Read the model definition and answer for the solid it produces. Units are mm, in the model's axes. Face numbers are marked on the shaded views. A direction names the side the tool comes from. Coordinates: 2 decimals unless noted, no trailing zeros. Order: outer loops, then holes, each group sorted by start corner. A loop starts at its lowest first (then second) coordinate and runs counter-clockwise, first axis right, second up. Notation, with made-up numbers: (-10, -2.5) - (42, -2.5) arc R14 cw to (42, 12.5) - close; hole circle Ø6 at (14, -19). An arc over 180 degrees is marked (long way). Use one line per item in the form item = value.
```python
from build123d import *

# Parameters (mm, degrees)
F0_W     = 40
F0_H     = 26
F1_DEPTH = 17
F2_T     = -1.5
F3_W     = 37
F3_H     = 8.5
F4_DEPTH = 2
F5_W     = 8.4
F5_H     = 3.5
F6_DEPTH = 1.5
F7_SIZE  = 2
F8_R     = 5


with BuildPart() as f1:
    # F0 (on Top) → F1 (new body)
    with BuildSketch(Plane.XY):
        Rectangle(F0_W, F0_H)
    extrude(amount=F1_DEPTH)

    # F2
    f2_openings = [f1.faces().sort_by_distance(p)[0] for p in [
        (0, 0, 17),
    ]]
    offset(amount=F2_T, openings=f2_openings)

    # F3 (on face) → F4 (join)
    with BuildSketch(Plane.XY.offset(1.5)):
        Rectangle(F3_W, F3_H)
    extrude(amount=F4_DEPTH)

    # F5 (on face) → F6 (cut, through all)
    with BuildSketch(Plane.YZ.offset(20)):
        with Locations((0, 5.25)):
            Rectangle(F5_W, F5_H)
    extrude(amount=-F6_DEPTH, mode=Mode.SUBTRACT)

    # F7
    f7_edges = [f1.edges().sort_by_distance(p)[0] for p in [
        (-18.5, 11.5, 9.25),
        (18.5, 11.5, 9.25),
        (18.5, -11.5, 9.25),
        (-18.5, -11.5, 9.25),
    ]]
    chamfer(f7_edges, length=F7_SIZE)

    # F8
    f8_edges = [f1.edges().sort_by_distance(p)[0] for p in [
        (-20, 13, 8.5),
        (20, 13, 8.5),
        (20, -13, 8.5),
        (-20, -13, 8.5),
    ]]
    fillet(f8_edges, radius=F8_R)


solid = f1.part
```
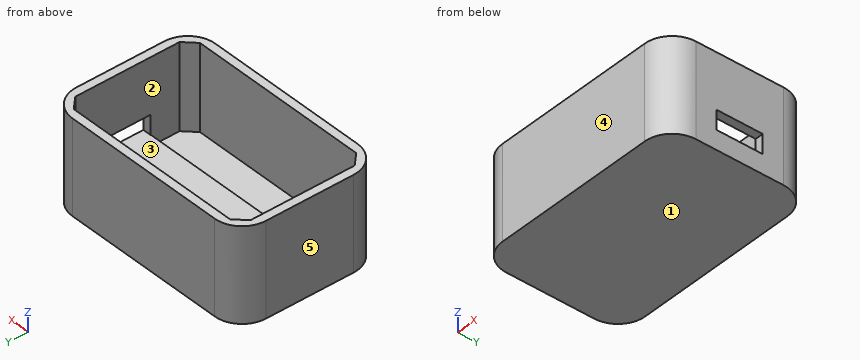
(1) Section D-D, the plane x = 7 is taken. Write down the section's boundary in (y, z).
Answer list:
outline = (-13, 0) - (13, 0) - (13, 17) - (11.5, 17) - (11.5, 1.5) - (4.25, 1.5) - (4.25, 3.5) - (-4.25, 3.5) - (-4.25, 1.5) - (-11.5, 1.5) - (-11.5, 17) - (-13, 17) - close
(2) Given pin 1 Ø1.5 at (x, y) = (13, 3.5) entering from +Z; pin 2 Ø3.5 at (x, y) = (9, -9) entering from +Z; pin 3 Ø1.2 at (x, z) = (19, 5) entering from +Y, each flat-ended and moving along its own axis, determine where each tip first touches the part or whether it passes through.
Answer list:
pin_1 = 3.5
pin_2 = 1.5
pin_3 = 11.67
(3) Section A-A, the plane y = -2.5 is taken. Write down the section's boundary in (x, z).
Answer list:
outline = (-20, 0) - (20, 0) - (20, 3.5) - (-18.5, 3.5) - (-18.5, 17) - (-20, 17) - close; (18.5, 7) - (20, 7) - (20, 17) - (18.5, 17) - close
(4) Section C-C, the plane z = 5.75 is taken. Write down the section's boundary in (x, y).
Answer list:
outline = (-20, -8) arc R5 ccw to (-15, -13) - (15, -13) arc R5 ccw to (20, -8) - (20, -4.2) - (18.5, -4.2) - (18.5, -9.5) - (16.5, -11.5) - (-16.5, -11.5) - (-18.5, -9.5) - (-18.5, 9.5) - (-16.5, 11.5) - (16.5, 11.5) - (18.5, 9.5) - (18.5, 4.2) - (20, 4.2) - (20, 8) arc R5 ccw to (15, 13) - (-15, 13) arc R5 ccw to (-20, 8) - close
(5) Which of the six approach directions +Z, -Z, +X, -X, +Y, -Y give full straight-line access (tool end or side, diameter ignored) to the marked faces 1 and 2?
Answer list:
face_1 = -Z, +X, -X, +Y, -Y
face_2 = +Z
(6) Section B-B, the plane z = 12.75 is taken. Write down the section's boundary in (x, y).
Answer list:
outline = (-20, -8) arc R5 ccw to (-15, -13) - (15, -13) arc R5 ccw to (20, -8) - (20, 8) arc R5 ccw to (15, 13) - (-15, 13) arc R5 ccw to (-20, 8) - close; hole (-18.5, -9.5) - (-16.5, -11.5) - (16.5, -11.5) - (18.5, -9.5) - (18.5, 9.5) - (16.5, 11.5) - (-16.5, 11.5) - (-18.5, 9.5) - close
(7) The mould has two halves that part along Y. Classify the marked faces 3, 4 and 5: +Y half, -Y half, draft (parallel to the pull), parting line (faces both ways), or undercut.
Answer list:
face_3 = undercut
face_4 = -Y half
face_5 = draft
(8) Straight lines are drawn through the part: L1, parallel to Y at x = 5, z = 2.75; L2, parallel to Y at x = -3.5, z = 10; L3, parallel to X at y = 7.5, z = 14. For each, find the intervals that lie inside material, in ascending order.
Answer list:
L1 = -13 to -11.5, -4.25 to 4.25, 11.5 to 13
L2 = -13 to -11.5, 11.5 to 13
L3 = -20 to -18.5, 18.5 to 20
